from build123d import *

# Parameters (mm, degrees)
SKETCH_2_R      = 2.1
EXTRUDE_1_DEPTH = 1


with BuildPart() as part:
    # 草图1 → 旋转1 (revolve)
    with BuildSketch(Plane.XY):
        with BuildLine():
            Line((14.944585174, 15.701905636), (0, 15.701905636))
            Line((0, 15.701905636), (0, -3.298094364))
            add(Edge.make_bspline(
                [(0, -3.298094364), (0.706455528, -3.332616299), (1.691072276, -3.219064863), (2.773175522, -2.870028275), (3.305020932, -2.665292125), (3.682415706, -2.517038895), (4.050641345, -2.355189766), (4.416695399, -2.20481684), (4.77817462, -2.003706717), (5.099926424, -1.754542973), (5.469244366, -1.550129904), (5.861768452, -1.245065409), (6.265016456, -0.923290365), (6.630974372, -0.544071897), (6.924875069, -0.139959882), (7.370604687, 0.048686033), (7.772218261, 0.161143877), (8.158981876, 0.24790247), (8.578399204, 0.358534367), (9.10951982, 0.547037122), (9.69818302, 0.72066457), (10.259773085, 0.91104592), (10.747610732, 1.028094825), (11.160281011, 1.214814977), (11.564815316, 1.481178609), (12.000197559, 1.680416472), (12.456348878, 1.97889325), (12.887671936, 2.339764988), (13.291414369, 2.770380198), (13.622058348, 3.171561468), (13.87545394, 3.574212032), (14.104629888, 3.983119622), (14.24807752, 4.50808303), (14.453255803, 4.977984441), (14.55328951, 5.613547364), (14.688797752, 6.352898821), (14.744580933, 7.850347198), (14.739662401, 9.917386792), (14.610748365, 12.725417472), (14.745577946, 14.655065366), (14.944585174, 15.701905636)],
                knots=[0, 0, 0, 0, 0.074980327, 0.104145363, 0.120682551, 0.135565386, 0.147239076, 0.163438876, 0.177614949, 0.191043322, 0.206610736, 0.222342481, 0.243822524, 0.261329251, 0.278460385, 0.295787667, 0.311179453, 0.323053348, 0.337863831, 0.357273022, 0.382918323, 0.403098398, 0.420289185, 0.436132056, 0.450933537, 0.471701704, 0.4868637, 0.508750883, 0.531302671, 0.549552014, 0.563884853, 0.581874699, 0.599060538, 0.621525796, 0.636019375, 0.667207468, 0.701413253, 0.794955071, 0.88706401, 1, 1, 1, 1], degree=3))
        make_face()
    revolve(axis=Axis((0, -3.298094364, 0), (0, 1, 0)))

    # 草图2 → 凸台-拉伸1 (add)
    with BuildSketch(Plane(origin=(0, 15.701905636, 0), x_dir=(1, 0, 0), z_dir=(0, 1, 0))):
        with BuildLine():
            Line((9.220360825, 12.953568862), (22.096520619, 3.788307875))
            ThreePointArc((22.096520619, 3.788307875), (24.05, 0), (22.096520619, -3.788307875))
            Line((22.096520619, -3.788307875), (9.220360825, -12.953568862))
            ThreePointArc((9.220360825, -12.953568862), (0, -15.9), (-9.220360825, -12.953568862))
            Line((-9.220360825, -12.953568862), (-22.096520619, -3.788307875))
            ThreePointArc((-22.096520619, -3.788307875), (-24.05, 0), (-22.096520619, 3.788307875))
            Line((-22.096520619, 3.788307875), (-9.220360825, 12.953568862))
            ThreePointArc((-9.220360825, 12.953568862), (0, 15.9), (9.220360825, 12.953568862))
        make_face()
        with Locations((19.4, 0)):
            Circle(SKETCH_2_R, mode=Mode.SUBTRACT)
        with Locations((-19.4, 0)):
            Circle(SKETCH_2_R, mode=Mode.SUBTRACT)
    extrude(amount=-EXTRUDE_1_DEPTH)


solid = part.part
Work out the finished part from the listing and answer in its coordinate system (mm). A direction names the side the tool comes from. Round coordinates to 2 decimals unless told otherwise and drop trailing zeros. Order: outer loops, then holes, each group sorted by start corner. A loop starts at its lowest first (then second) coordinate and runs counter-clockwise, first axis right, second up. Notation, with made-up numbers: M 26,31.5 L 50,31.5 A10 cw 50,47.5 Z; hole C -15,-22 d10. An arc over 180 degrees is marked long. Put each result on its own line as item: value. Start each with the question number.
Q1. For a pull along Z with two mould halves and no side action, classify faces 3 (the cylindrical face through (-17.397, 15.209, -0.631)), 4 (the flat face through (-15.749, 15.209, -8.307)), 5 (the cylindrical face through (-24.05, 15.21, 0.06)), 6 (the cylindrical face through (21.403, 15.209, -0.631)) as pulls with the +Z half, pulls with the -Z half, needs draft (parallel to the pull), parting line crosses it, or undercut.
Q2. Flat-ended cylindrical pins translate along their axes: pin 1 (1.5 mm diameter, centred on x = -11.5, y = 4.5, fed in from +Z); pin 2 (1.5 mm diameter, centred on y = 7.5, z = 5, fed in from -X); pin 3 (6 mm diameter, centred on y = 1.5, z = -11, fed in from -X); pin 4 (4 mm diameter, centred on x = -19.4, z = 0, fed in from -Y). Find the tip coordinate at first contact, or state that the pin passes through.
Q3. A tool of negligible diameter and unlimited length cuts with its end or side. For faces 1 (the flat face through (-15.568, 15.209, 8.435)), 2 (the flat face through (-11, 14.702, 11)), from which of +Z, -Z, +X, -X, +Y, -Y can it reach the whole face along a straight path? Write none if from no direction.
Q4. Straight lines are drawn through the part: L1, parallel to Z at x = -19.4, y = 15.45; L2, parallel to Y at x = 10.5, z = -2; L3, parallel to X at y = 3.25, z = 10. For each, find the intervals that lie inside material, in ascending order. Write a range as [from, to].
Q5. Section A-A, the plane x = 19.4 is taken. Write down the section's boundary in (y, z), and give its area (3 significant figures).
Findings below:
1. face 3: undercut
1. face 4: pulls with the -Z half
1. face 5: parting line crosses it
1. face 6: undercut
2. pin 1: stops at z = 9.47
2. pin 2: stops at x = -14.1
2. pin 3: stops at x = -10.7
2. pin 4: passes through
3. face 1: +Z, -X, +Y, -Y
3. face 2: -Y
4. L1: z = [-5.71, -2.1], [2.1, 5.71]
4. L2: y = [1.02, 15.7]
4. L3: x = [-9.31, 9.31]
5. outline: M 14.7,-5.71 L 15.7,-5.71 L 15.7,-2.1 L 14.7,-2.1 Z; M 14.7,2.1 L 15.7,2.1 L 15.7,5.71 L 14.7,5.71 Z
5. area: 7.22 mm^2
